Input: part model. Units: mm. Frame: model coordinates. A direction names the side the tool comes from. Give positions to 0.01 mm unless a question says otherwise; leave off trailing zeros. Loops run counter-clockwise (first coordinate to the right, second up) from the corner with the lowest first, then second, coordinate; pieces in that order, holes last. Notation, with made-up numbers: (49, 53.25) -> (56, 53.25) arc R6 ccw to (56, 57.25) -> close; hole circle Ø7 at (-27.75, 67.5). An arc over 180 degrees is marked (long way). Answer as a JSON object with one key per item and string values.
Autodesk Inventor part; units mm, degrees
ref_plane "YZ Plane" through (0, 0, 0) normal (1, 0, 0) x (0, 1, 0)
ref_plane "XZ Plane" through (0, 0, 0) normal (0, 1, 0) x (-1, 0, 0)
ref_plane "XY Plane" through (0, 0, 0) normal (0, 0, 1) x (1, 0, 0)
sketch "Sketch1" plane through (0, 0, 0) normal (0, 0, 1) x (1, 0, 0)
  circle A0 centre (0, 0) radius 50 construction
  circle A1 centre (0, 0) radius 52.5
  dimension "d0" = 100
  dimension "d1" = 105
extrude "Extrusion1" add sketch "Sketch1" along normal blind 1.5
sketch "Sketch2" plane through (0, 0, 1.5) normal (0, 0, 1) x (1, 0, 0)
  line L0 (-20, -20) -> (20, -20) construction
  line L1 (20, -20) -> (20, 20) construction
  line L2 (20, 20) -> (-20, 20) construction
  line L3 (-20, 20) -> (-20, -20) construction
  line L4 (-20, -20) -> (20, 20) construction
  line L5 (20, -20) -> (-20, 20) construction
  circle A0 centre (-20, 20) radius 22.5
  circle A1 centre (20, 20) radius 22.5
  circle A2 centre (20, -20) radius 22.5
  circle A3 centre (-20, -20) radius 22.5
  circle A4 centre (0, 0) radius 52.5
  point P0 (-9.6922, 0)
  point P1 (0, -9.6922)
  point P2 (9.6922, 0)
  point P3 (0, 9.6922)
  point P4 (0, -30.3078)
  point P5 (-30.3078, 0)
  point P6 (0, 30.3078)
  point P7 (30.3078, 0)
  dimension "d4" = 45
  dimension "d5" = 40
extrude "Extrusion2" add sketch "Sketch2" along normal blind 8 contours A1 A2 A3 A0 | A4
sketch "Sketch3" plane through (0, 0, 9.5) normal (0, 0, 1) x (1, 0, 0)
  circle A0 centre (0, 0) radius 51
  circle A1 centre (0, 0) radius 52.5
  dimension "d8" = 1.5
extrude "Extrusion3" add sketch "Sketch3" along normal blind 18
sketch "Sketch4" plane through (0, 0, 0) normal (0, 0, -1) x (-1, 0, 0)
  line L0 (0, 0) -> (42, 0) construction
  circle A0 centre (42, 0) radius 6
  circle A1 centre (0, 42) radius 6
  circle A2 centre (-42, 0) radius 6
  circle A3 centre (0, -42) radius 6
  dimension "d11" = 12
  dimension "d12" = 42
  dimension "d15" = 360
extrude "Extrusion4" cut sketch "Sketch4" against normal blind 2
properties part number "Base"
Q1. Section C-C, the plane y = 20. Return the cut outline in (x, z).
Evaluation:
{"outline": "(-48.54, 0) -> (48.54, 0) -> (48.54, 27.5) -> (46.91, 27.5) -> (46.91, 9.5) -> (42.5, 9.5) -> (42.5, 1.5) -> (-42.5, 1.5) -> (-42.5, 9.5) -> (-46.91, 9.5) -> (-46.91, 27.5) -> (-48.54, 27.5) -> close"}
Q2. Section A-A, the plane z = 7. Return the cut outline in (x, y), then the cut area to 3 significant figures.
Evaluation:
{"outline": "circle Ø105 at (0, 0); (-9.69, 0) arc R22.5 cw to (0, -9.69) arc R22.5 cw to (9.69, 0) arc R22.5 cw to (0, 9.69) arc R22.5 cw to start; hole (-30.31, 0) arc R22.5 ccw (long way) to (0, -30.31) arc R22.5 ccw (long way) to (30.31, 0) arc R22.5 ccw (long way) to (0, 30.31) arc R22.5 ccw (long way) to start", "area": "2,580 mm2"}
Q3. Ray query, line 1 along Y through (x, z) = (0, 0.65); line 2 along Y through (x, z) = (0, 16.75); line 3 along X through (y, z) = (31, 1.75). Return the intervals inside material, ascending.
Evaluation:
{"line 1": "y = -52.5 to -48, -36 to 36, 48 to 52.5", "line 2": "y = -52.5 to -51, 51 to 52.5", "line 3": "x = -42.37 to -39.63, -0.37 to 0.37, 39.63 to 42.37"}
Q4. Draft query along Y for faces 1 (the flat face through (42, 0, 2)), 2 (the cylindrical face through (50.076, -15.77, 13.558)), 3 (the cylindrical face through (-4.02, 4.16, 5.44)), 4 (the flat face through (-8, 51, 27.5)). Return one class per face: +Y half, -Y half, draft (parallel to the pull), parting line (faces both ways), or undercut.
Evaluation:
{"face 1": "undercut", "face 2": "parting line", "face 3": "undercut", "face 4": "draft"}
Q5. Section B-B, the plane x = -23. Return the cut outline in (y, z).
Evaluation:
{"outline": "(-47.19, 0) -> (47.19, 0) -> (47.19, 27.5) -> (45.52, 27.5) -> (45.52, 9.5) -> (42.3, 9.5) -> (42.3, 1.5) -> (-42.3, 1.5) -> (-42.3, 9.5) -> (-45.52, 9.5) -> (-45.52, 27.5) -> (-47.19, 27.5) -> close"}
Q6. Pin query (flat end, axial travel): pin 1 (1.5 mm diameter, centred on y = 2, z = 11, fed in from -X); pin 2 (13 mm diameter, centred on x = -2, y = 40, fed in from -Z); pin 3 (10 mm diameter, centred on x = -40, z = 13, fed in from +Y); pin 4 (6 mm diameter, centred on y = 8, z = 24.5, fed in from -X). Return the tip coordinate at first contact, or that it passes through.
Evaluation:
{"pin 1": "stops at x = -52.49", "pin 2": "stops at z = 0", "pin 3": "stops at y = 39.13", "pin 4": "stops at x = -52.26"}
Q7. Section D-D, the plane z = 16.75. Return the cut outline in (x, y), then the cut area to 3 significant figures.
Evaluation:
{"outline": "circle Ø105 at (0, 0); hole circle Ø102 at (0, 0)", "area": "488 mm2"}
Q8. Access query for faces 5 (the cylindrical face through (-11.056, 49.787, 18.374)), 6 (the flat face through (-1, 1, 0)), 7 (the flat face through (0, 42, 2)). Directions: +Z, -Z, +X, -X, +Y, -Y. A direction counts if a zero-diameter tool reaches every point of the face in a straight line with its end or side. Return the directions, or none.
Evaluation:
{"face 5": "+Z", "face 6": "-Z, +X, -X, +Y, -Y", "face 7": "-Z"}
